Verification items for this drawing (mm, ordinates from the low corner). Coordinates: 2 decimals unless noted, no trailing zeros. Order: outer loops, then holes, each group sorted by start corner. A loop starts at its lowest first (then second) coordinate and runs counter-clockwise, first axis right, second up. Notation, with made-up numbers: M -8,-3.75 L 41,-3.75 A12 ccw 41,12.25 Z; hole C 24.25,65 d6. An arc over 180 degrees is marked long. One line per item, written item: value. Start each with the question number.
1) Sectioned sample at C-C, the plane x = 6. Enter the section's corners in (y, z).
2) Sectioned sample at A-A, the plane z = 16.5. Enter the section's corners in (x, y).
3) Sectioned sample at D-D, the plane z = 2.5. Enter the section's corners in (x, y).
4) Draft check along Y on the marked faces 1, 2 and 3. Enter one of: pulls with the +Y half, pulls with the -Y half, needs draft (parallel to the pull), parting line crosses it, or undercut.
5) Thickness scan on L1, parallel to Y at x = 6, z = 13.5; L2, parallel to X at y = 22.7, z = 3.5; L3, parallel to X at y = 24.5, z = 9. Record the ranges inside material, lowest first. Write a range as from..to.
6) Sectioned sample at B-B, the plane y = 4.7. Enter the section's corners in (x, z).
7) Go/stop test with a flat-tipped pin: P1, Ø1.5, axis at y = 14.5, z = 4.5, coming from the -X side. Record where the tip stops, or that it passes through.
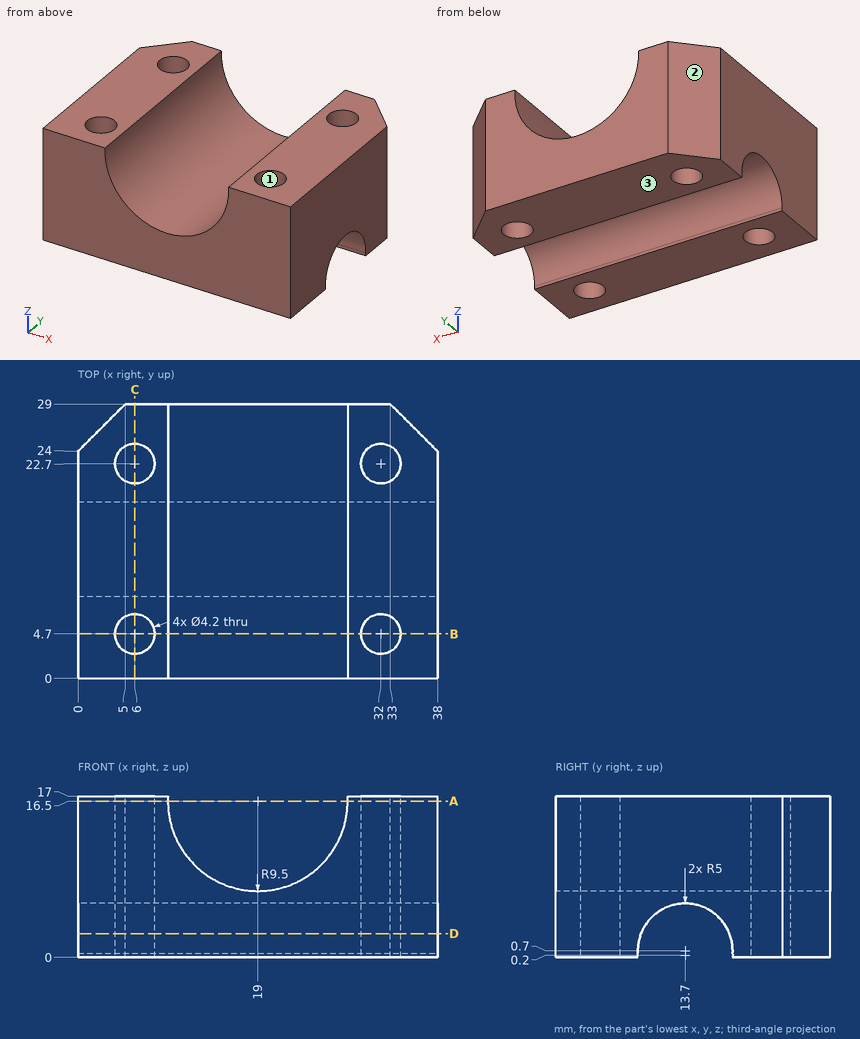
Final values:
1. outline: M 0,0 L 2.6,0 L 2.6,17 L 0,17 Z; M 6.8,0 L 8.7,0 A5 cw 8.71,0.45 A5 cw long 18.69,0.45 A5 cw 18.7,0 L 20.6,0 L 20.6,17 L 6.8,17 Z; M 24.8,0 L 29,0 L 29,17 L 24.8,17 Z
2. outline: M 0,0 L 9.5,0 L 9.5,29 L 5,29 L 0,24 Z; M 28.5,0 L 38,0 L 38,24 L 33,29 L 28.5,29 Z; hole C 6,4.7 d4.2; hole C 6,22.7 d4.2; hole C 32,4.7 d4.2; hole C 32,22.7 d4.2
3. outline: M 0,0 L 38,0 L 38,9.04 L 0,9.04 Z; M 0,18.36 L 38,18.36 L 38,24 L 33,29 L 5,29 L 0,24 Z; hole C 6,4.7 d4.2; hole C 6,22.7 d4.2; hole C 32,4.7 d4.2; hole C 32,22.7 d4.2
4. face 1: undercut
4. face 2: pulls with the +Y half
4. face 3: needs draft
5. L1: y = 0..2.6, 6.8..20.6, 24.8..29
5. L2: x = 0..3.9, 8.1..29.9, 34.1..38
5. L3: x = 0.5..4.92, 7.08..13.17, 24.83..30.92, 33.08..37.5
6. outline: M 0,0 L 3.9,0 L 3.9,17 L 0,17 Z; M 8.1,0 L 29.9,0 L 29.9,17 L 28.49,17 A9.5 cw long 9.51,17 L 8.1,17 Z; M 34.1,0 L 38,0 L 38,17 L 34.1,17 Z
7. P1: passes through
